Study the drawing (mm; zero at the part's minimum x, y, z) and answer. A direction names the side the tool comes from. Give positions to 0.01 mm unless a question says otherwise; leave off trailing zeros. Write each loop counter-clockwise with the first axis right and the second up, starting at its lowest first coordinate (ties: lowest second). Pieces come first, ordered by that corner, then holes. Notation, with made-up numbers: (-38.5, -11) - (-3.5, -11) arc R30 cw to (-3.5, 21) - close; hole circle Ø11 at (-36.5, 18). An arc over 180 degrees is marked (long way). Write each question's results on one line, items separated by ' | '. Start each with the question number.
Q1. For the marked faces 1, 2, 3, 4 and 5, determine the directions among +Z, -Z, +X, -X, +Y, -Y from which every point of the face is accessible in a straight line to the end or side of a thin tool.
Q2. Section D-D (y = 4.25) is taken. Determine the outline of the cut face in (x, z) (3 decimals).
Q3. Section B-B (z = 7.5) is taken. Determine the outline of the cut face in (x, y), plus the area to 3 significant figures.
Q4. Section C-C (x = 45) is taken. Determine the outline of the cut face in (y, z) (3 decimals).
Q5. Section A-A (y = 14.5) is taken. Determine the outline of the cut face in (x, z) (3 decimals).
Q6. For a pull along X with two mould halves and no side action, classify the marked faces 6, 7 and 8 as pulls with the +X half, pulls with the -X half, needs draft (parallel to the pull), parting line crosses it, or undercut.
Q7. Find the intervals of material crossed by probe 1 along X at (y, z) = (10.75, 8.5); probe 2 along Y at (x, z) = (43.5, 17); probe 3 along X at (y, z) = (5.5, 12), in increasing order.
Q8. Flat-ended cylindrical pins translate along their axes: pin 1 Ø6.5 at (x, z) = (6.5, 20.5) entering from -Y; pin 2 Ø1 at (y, z) = (12, 18.5) entering from +X; pin 3 Ø7 at (y, z) = (8.5, 2.5) entering from -X. Find the tip coordinate at first contact, or state that the pin passes through.
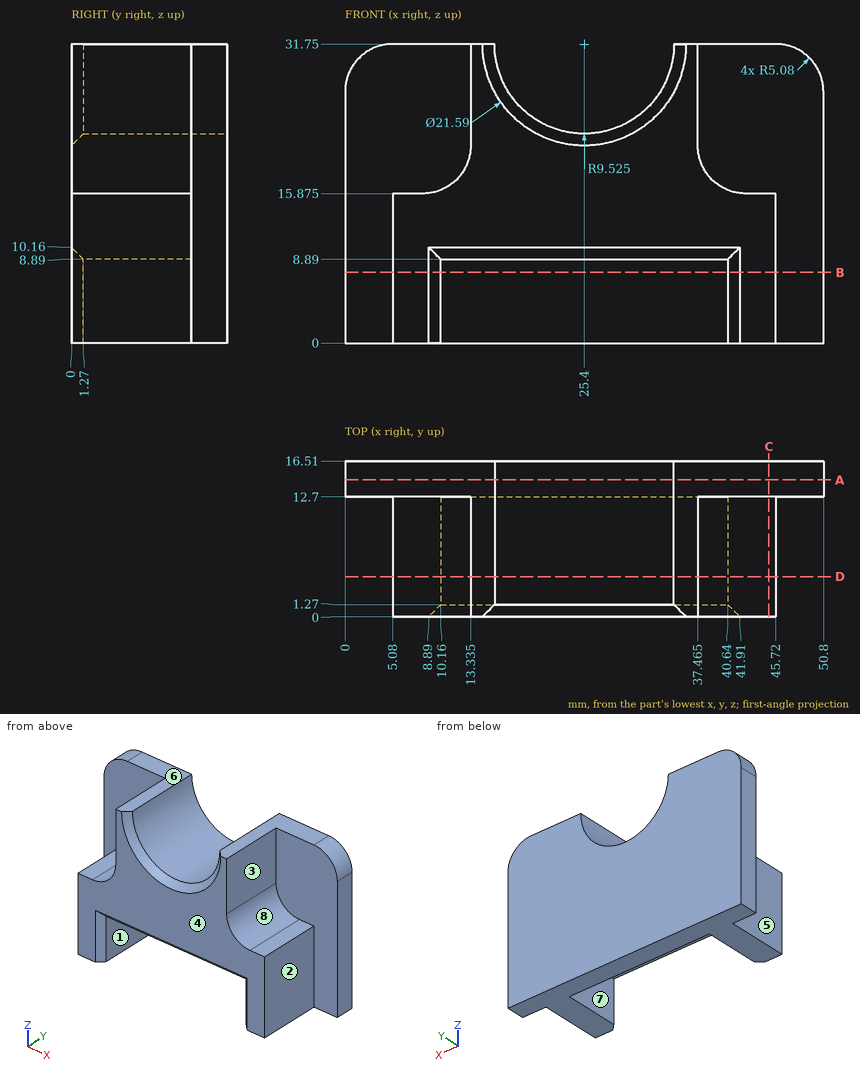
Answers below:
1) face 1: -Z, -Y | face 2: +Z, -Z, +X, -Y | face 3: +Z, +X, -Y | face 4: +Z, -Z, +X, -X, -Y | face 5: +Z, -Z, -X, -Y
2) outline: (5.08, 0) - (10.16, 0) - (10.16, 8.89) - (40.64, 8.89) - (40.64, 0) - (45.72, 0) - (45.72, 15.875) - (42.545, 15.875) arc R5.08 cw to (37.465, 20.955) - (37.465, 31.75) - (34.925, 31.75) arc R9.525 cw to (15.875, 31.75) - (13.335, 31.75) - (13.335, 20.955) arc R5.08 cw to (8.255, 15.875) - (5.08, 15.875) - close
3) outline: (0, 12.7) - (5.08, 12.7) - (5.08, 0) - (8.89, 0) - (10.16, 1.27) - (10.16, 12.7) - (40.64, 12.7) - (40.64, 1.27) - (41.91, 0) - (45.72, 0) - (45.72, 12.7) - (50.8, 12.7) - (50.8, 16.51) - (0, 16.51) - close | area: 321 mm2
4) outline: (0, 0) - (16.51, 0) - (16.51, 31.75) - (12.7, 31.75) - (12.7, 15.875) - (0, 15.875) - close
5) outline: (0, 0) - (50.8, 0) - (50.8, 26.67) arc R5.08 ccw to (45.72, 31.75) - (34.925, 31.75) arc R9.525 cw to (15.875, 31.75) - (5.08, 31.75) arc R5.08 ccw to (0, 26.67) - close
6) face 6: needs draft | face 7: undercut | face 8: pulls with the +X half
7) probe 1: x = 5.08 to 10.16, 40.64 to 45.72 | probe 2: y = 12.7 to 16.51 | probe 3: x = 5.08 to 45.72
8) pin 1: stops at y = 12.7 | pin 2: stops at x = 38.41 | pin 3: stops at x = 5.08
